Autodesk Inventor part; units mm, degrees
ref_plane "YZ Plane" through (0, 0, 0) normal (1, 0, 0) x (0, 1, 0)
ref_plane "XZ Plane" through (0, 0, 0) normal (0, 1, 0) x (-1, 0, 0)
ref_plane "XY Plane" through (0, 0, 0) normal (0, 0, 1) x (1, 0, 0)
sketch "Sketch1" plane through (0, 0, 0) normal (1, 0, 0) x (0, 1, 0)
  line L0 (32.5, 9) -> (-32.5, 9)
  line L1 (-32.5, 9) -> (-32.5, -9)
  line L2 (-32.5, -9) -> (32.5, -9)
  line L3 (32.5, -9) -> (32.5, 9)
  line L4 (32.5, 9) -> (-32.5, -9) construction
  line L5 (-32.5, 9) -> (32.5, -9) construction
  circle A0 centre (-25, 0) radius 3
  circle A1 centre (25, 0) radius 3
  line L6 (-10, -5) -> (-10, 5) construction
  line L7 (-13, -5) -> (-13, 5)
  line L8 (-7, 5) -> (-7, -5)
  arc A2 (-13, -5) -> (-7, -5) centre (-10, -5) ccw
  arc A3 (-7, 5) -> (-13, 5) centre (-10, 5) ccw
  line L9 (10, -5) -> (10, 5) construction
  line L10 (13, -5) -> (13, 5)
  line L11 (7, 5) -> (7, -5)
  arc A4 (7, -5) -> (13, -5) centre (10, -5) ccw
  arc A5 (13, 5) -> (7, 5) centre (10, 5) ccw
  point P0 (0, 0)
  point P1 (-10, 0)
  point P2 (10, 0)
  dimension "d0" = 25
  dimension "d1" = 50
  dimension "d2" = 65
  dimension "d3" = 6
  dimension "d4" = 10
  dimension "d5" = 20
  dimension "d6" = 10
  dimension "d7" = 3
  dimension "d8" = 18
extrude "Extrusion1" add sketch "Sketch1" along normal blind 12
sketch "Sketch2" plane through (0, 0, 0) normal (-1, 0, 0) x (0, 0, 1)
  line L0 (9, -32.5) -> (-9, -32.5)
  line L1 (9, 32.5) -> (9, -32.5)
  line L2 (-9, 32.5) -> (9, 32.5)
  line L3 (-9, -32.5) -> (-9, 32.5)
  circle A0 centre (0, -25) radius 3
  circle A1 centre (0, 25) radius 3
  arc A2 (-5, 13) -> (-5, 7) centre (-5, 10) ccw
  line L4 (5, 13) -> (-5, 13)
  arc A3 (5, 7) -> (5, 13) centre (5, 10) ccw
  line L5 (-5, 7) -> (5, 7)
  line L6 (5, -7) -> (-5, -7)
  arc A4 (5, -13) -> (5, -7) centre (5, -10) ccw
  line L7 (-5, -13) -> (5, -13)
  arc A5 (-5, -7) -> (-5, -13) centre (-5, -10) ccw
  line L8 (5, 10) -> (-5, 10) construction
  line L9 (5, 8.25) -> (-5, 8.25)
  line L10 (-5, 11.75) -> (5, 11.75)
  arc A6 (5, 8.25) -> (5, 11.75) centre (5, 10) ccw
  arc A7 (-5, 11.75) -> (-5, 8.25) centre (-5, 10) ccw
  line L11 (5, -10) -> (-5, -10) construction
  line L12 (5, -11.75) -> (-5, -11.75)
  line L13 (-5, -8.25) -> (5, -8.25)
  arc A8 (5, -11.75) -> (5, -8.25) centre (5, -10) ccw
  arc A9 (-5, -8.25) -> (-5, -11.75) centre (-5, -10) ccw
  point P0 (0, 0)
  point P1 (0, 10)
  point P2 (0, -10)
  dimension "d11" = 3.5
extrude "Extrusion2" add sketch "Sketch2" against normal blind 3 contours L4 A3 L5 A2 | A4 L7 A5 L6
chamfer "Chamfer1" distance 5 angle 45 4 edges at (6, -32.5, 9) (6, -32.5, -9) (6, 32.5, -9) (6, 32.5, 9)
sketch "Sketch3" plane through (0, -27.5, 9) normal (0, 0, 1) x (1, 0, 0)
  line L0 (0, 55) -> (12, 55)
  line L1 (0, 55) -> (0, 0)
  line L2 (12, 0) -> (0, 0)
  line L3 (12, 55) -> (12, 0)
  line L4 (12, 10) -> (8.5, 10)
  line L5 (8.5, 10) -> (8.5, 45)
  line L6 (8.5, 45) -> (12, 45)
  line L7 (12, 45) -> (12, 10)
  line L8 (12, 10) -> (8.5, 45) construction
  line L9 (8.5, 10) -> (12, 45) construction
  point P0 (0, 27.5)
  point P1 (10.25, 27.5)
  point P2 (0, 27.5)
  point P3 (12, 10)
  dimension "d17" = 35
  dimension "d18" = 3.5
extrude "Extrusion3" cut sketch "Sketch3" against normal through all contours L3 L4 L5 L6
equation "\"d1\" = 2 * d0"
properties part number "ToolDock_Center" material "ABS Plastic"
Can you work these out from the model? Positions are in its coordinate system, mm. A direction names the side the tool comes from. Coordinates: 2 decimals unless noted, no trailing zeros. Loops run counter-clockwise (first coordinate to the right, second up) from the corner with the lowest first, then second, coordinate; pieces in that order, holes last. Notation, with made-up numbers: M 4,32.5 L 19,32.5 A23 ccw 19,43.5 Z; hole C 58,-14.75 d6. An arc over 180 degrees is marked long. Put each result on its own line as item: value. Start each with the question number.
(1) I need wall thicknesses on probe 1 along Y at (x, z) = (7, 3.5); probe 2 along Z at (x, y) = (3, -25); probe 3 along Y at (x, z) = (5.25, -2). Which ranges of each line are inside material? Lowest first, please.
(2) Imagine slicing it at A-A on y = -10. List the corners of the cut face in (x, z) for me.
(3) Will these pins go through, and if not, where does the flat tip stop? pin 1 Ø1.5 at (x, z) = (2.5, -6) entering from +Y; pin 2 Ø5.5 at (y, z) = (5.5, 4) entering from +X; pin 3 Ø3.5 at (y, z) = (-25, 0) entering from -X; pin 4 Ø3 at (y, z) = (10.5, -3.5) entering from +X.
(4) Imagine slicing it at D-D on y = 25. List the corners of the cut face in (x, z) for me, and give its area (3 significant figures).
(5) Imagine slicing it at C-C on z = 0. Give the number of separate pieces and of enclosed holes in the cut face, and give its area (4 significant figures).
(6) Which directions (+Z, -Z, +X, -X, +Y, -Y) give clear straight access to the entire face, cutting with the end or side of a thin tool? Please do faces 4 (the face through (10, -17.5, 0)), 5 (the face through (6, 10, 8)), 6 (the face through (1, -8.25, 0)), 7 (the face through (6, 32.5, 0)).
(7) Imagine slicing it at B-B on x = 2. List the corners of the cut face in (y, z) for me, and give its area (3 significant figures).
(8) We'd pull the mould along Y, two halves only. Please class faces 1 (the face through (6, 7, 0)), 2 (the face through (5.9, -30, -6.5)), 3 (the face through (5, 0, 9)): +Y half, -Y half, draft (parallel to the pull), parting line (faces both ways), or undercut.
Worked answers:
1. probe 1: y = -32.5 to -13, -7 to 7, 13 to 32.5
1. probe 2: z = -9 to -3, 3 to 9
1. probe 3: y = -32.5 to -27.24, -22.76 to -13, -7 to 7, 13 to 22.76, 27.24 to 32.5
2. outline: M 0,-9 L 8.5,-9 L 8.5,-8 L 3,-8 L 3,-6.75 L 0,-6.75 Z; M 0,6.75 L 3,6.75 L 3,8 L 8.5,8 L 8.5,9 L 0,9 Z
3. pin 1: stops at y = 31.25
3. pin 2: stops at x = 8.5
3. pin 3: passes through
3. pin 4: stops at x = 3
4. outline: M 0,-9 L 12,-9 L 12,-3 L 0,-3 Z; M 0,3 L 12,3 L 12,9 L 0,9 Z
4. area: 144 mm2
5. separate pieces: 5
5. enclosed holes: 0
5. area: 426.5 mm2
6. face 4: +Z, -Z, +X
6. face 5: +X
6. face 6: +X, -X
6. face 7: +Z, -Z, +X, -X, +Y
7. outline: M -32.5,-4 L -27.5,-9 L 27.5,-9 L 32.5,-4 L 32.5,4 L 27.5,9 L -27.5,9 L -32.5,4 Z; hole C -25,0 d6; hole M -11.75,-5 A1.75 ccw -8.25,-5 L -8.25,5 A1.75 ccw -11.75,5 Z; hole M 8.25,-5 A1.75 ccw 11.75,-5 L 11.75,5 A1.75 ccw 8.25,5 Z; hole C 25,0 d6
7. area: 974 mm2
8. face 1: undercut
8. face 2: -Y half
8. face 3: draft
